```python
from build123d import *

# Parameters (mm, degrees)
SKETCH1_W           = 40
SKETCH1_H           = 40
BOSS_EXTRUDE1_DEPTH = 90
SKETCH2_R           = 18.5
CUT_EXTRUDE1_DEPTH  = 45
SKETCH3_R           = 16.5
CUT_EXTRUDE2_DEPTH  = 41
SKETCH4_W           = 40
SKETCH4_H           = 40
CUT_EXTRUDE3_DEPTH  = 21
SKETCH6_W           = 20
SKETCH6_H           = 15
CUT_EXTRUDE4_DEPTH  = 83.225300243
SKETCH8_W           = 20
SKETCH8_H           = 15
CUT_EXTRUDE5_DEPTH  = 83.225300243
SKETCH11_W          = 40
SKETCH11_H          = 28.5
CUT_EXTRUDE8_DEPTH  = 83.225300243


with BuildPart() as part:
    # Sketch1 → Boss-Extrude1 (new body)
    with BuildSketch(Plane(origin=(0, 0, 0), x_dir=(1, 0, 0), z_dir=(0, 1, 0))):
        Rectangle(SKETCH1_W, SKETCH1_H)
    extrude(amount=BOSS_EXTRUDE1_DEPTH)

    # Sketch2 → Cut-Extrude1 (cut)
    with BuildSketch(Plane(origin=(0, 90, 0), x_dir=(1, 0, 0), z_dir=(0, 1, 0))):
        with Locations(Location((0, 0, 0), (0, 0, 270))):
            Circle(SKETCH2_R)
    extrude(amount=-CUT_EXTRUDE1_DEPTH, mode=Mode.SUBTRACT)

    # Sketch3 → Cut-Extrude2 (cut)
    with BuildSketch(Plane(origin=(0, 45, 0), x_dir=(1, 0, 0), z_dir=(0, 1, 0))):
        with Locations(Location((0, 0, 0), (0, 0, 270))):
            Circle(SKETCH3_R)
    extrude(amount=-CUT_EXTRUDE2_DEPTH, mode=Mode.SUBTRACT)

    # Sketch4 → Cut-Extrude3 (cut)
    with BuildSketch(Plane(origin=(0, 90, 0), x_dir=(1, 0, 0), z_dir=(0, 1, 0))):
        Rectangle(SKETCH4_W, SKETCH4_H)
    extrude(amount=-CUT_EXTRUDE3_DEPTH, mode=Mode.SUBTRACT)

    # Sketch6 → Cut-Extrude4 (cut, through all)
    with BuildSketch(Plane.XY.offset(20)):
        with Locations((0, 15)):
            Rectangle(SKETCH6_W, SKETCH6_H)
    extrude(amount=-CUT_EXTRUDE4_DEPTH, mode=Mode.SUBTRACT)

    # Sketch8 → Cut-Extrude5 (cut, through all)
    with BuildSketch(Plane.ZY.offset(20)):
        with Locations((0, 15)):
            Rectangle(SKETCH8_W, SKETCH8_H)
    extrude(amount=-CUT_EXTRUDE5_DEPTH, mode=Mode.SUBTRACT)

    # Sketch11 → Cut-Extrude8 (cut, through all)
    with BuildSketch(Plane.XY.offset(20)):
        with Locations((0, 14.25)):
            Rectangle(SKETCH11_W, SKETCH11_H)
    extrude(amount=-CUT_EXTRUDE8_DEPTH, mode=Mode.SUBTRACT)


solid = part.part
```
Part model, mm, in its own coordinate system. A direction names the side the tool comes from. Round coordinates to 2 decimals unless told otherwise and drop trailing zeros. Loops run counter-clockwise (first coordinate to the right, second up) from the corner with the lowest first, then second, coordinate; pieces in that order, holes last. Notation, with made-up numbers: (48.5, 20.5) -> (73.5, 20.5) arc R30 cw to (73.5, 53.5) -> close; hole circle Ø3 at (-16.75, 27.5). An arc over 180 degrees is marked (long way). Use one line per item in the form item = value. Start each with the question number.
Item 1: Tool access for faces 5 (the cylindrical face through (-7.086, 57.168, 17.089)), 6 (the flat face through (-13.4, 69, 13.2)): list every direction of +Z, -Z, +X, -X, +Y, -Y with a clear straight run to the whole face (end or side of a thin tool).
Item 2: Band-saw the part on D-D (z = 17.5). List the corners of the cut face in (x, y), plus the area to 3 significant figures.
Item 3: Band-saw the part on B-B (y = 53). List the corners of the cut face in (x, z), plus the area to 3 significant figures.
Item 4: Band-saw the part on A-A (x = 0). List the corners of the cut face in (y, z), plus the area to 4 significant figures.
Item 5: Band-saw the part on C-C (z = 0). List the corners of the cut face in (x, y), plus the area to 4 significant figures.
Item 6: Two-plate mould, pull along X, no slides. Class faces 1 (the flat face through (0, 45, -17)), 2 (the flat face through (-18, 28.5, 0)), 3 (the cylindrical face through (-16.108, 36.866, -3.577)), 4 (the flat face through (20, 48, 0)): released by +X, released by -X, zero draft, split by the parting line, or undercut.
Item 7: Drill centre lines: line 1 along X through (y, z) = (36, 0); line 2 along X through (y, z) = (53, 0); line 3 along Z through (x, y) = (11, 35). Where is each one in solid material? Low to high.
Data:
q1.face_5 = +Y
q1.face_6 = +Z, -Z, +X, -X, +Y
q2.outline = (-20, 28.5) -> (20, 28.5) -> (20, 69) -> (6, 69) -> (6, 45) -> (-6, 45) -> (-6, 69) -> (-20, 69) -> close
q2.area = 1,330 mm^2
q3.outline = (-20, -20) -> (20, -20) -> (20, 20) -> (-20, 20) -> close; hole circle Ø37 at (0, 0)
q3.area = 525 mm^2
q4.outline = (28.5, -20) -> (69, -20) -> (69, -18.5) -> (45, -18.5) -> (45, -16.5) -> (28.5, -16.5) -> close; (28.5, 16.5) -> (45, 16.5) -> (45, 18.5) -> (69, 18.5) -> (69, 20) -> (28.5, 20) -> close
q4.area = 187.5 mm^2
q5.outline = (-20, 28.5) -> (-16.5, 28.5) -> (-16.5, 45) -> (-18.5, 45) -> (-18.5, 69) -> (-20, 69) -> close; (16.5, 28.5) -> (20, 28.5) -> (20, 69) -> (18.5, 69) -> (18.5, 45) -> (16.5, 45) -> close
q5.area = 187.5 mm^2
q6.face_1 = undercut
q6.face_2 = zero draft
q6.face_3 = undercut
q6.face_4 = released by +X
q7.line_1 = -20 to -16.5, 16.5 to 20
q7.line_2 = -20 to -18.5, 18.5 to 20
q7.line_3 = -20 to -12.3, 12.3 to 20
